```python
from build123d import *

# Parameters (mm, degrees)
F0_R     = 5
F1_DEPTH = 10
F2_SIZE  = 0.5
F4_D     = 9


with BuildPart() as f1:
    # F0 (on Front) → F1 (new body, symmetric)
    with BuildSketch(Plane.XZ):
        Polygon((18, 18), (0, 18), (-18, 18), (-18, -1), (-35, -1), (-35, -25), (0, -25), (35, -25), (35, -1), (18, -1), align=None)
        Circle(F0_R, mode=Mode.SUBTRACT)
    extrude(amount=F1_DEPTH, both=True)

    # F2
    f2_edges = [f1.edges().sort_by_distance(p)[0] for p in [
        (0, 10, 18),
        (-18, 0, 18),
        (0, -10, 18),
        (18, 0, 18),
        (-18, 0, -1),
        (-26.5, 10, -1),
        (-35, 0, -1),
        (-26.5, -10, -1),
        (-18, 10, 8.5),
        (-18, -10, 8.5),
        (-35, 10, -13),
        (-35, 0, -25),
        (-35, -10, -13),
        (35, 0, -25),
        (35, 10, -13),
        (35, 0, -1),
        (35, -10, -13),
        (18, 10, 8.5),
        (18, -10, 8.5),
        (18, 0, -1),
        (26.5, 10, -1),
        (26.5, -10, -1),
        (0, 10, -25),
        (0, -10, -25),
    ]]
    chamfer(f2_edges, length=F2_SIZE)

    # F4 (through all)
    with Locations(Plane(origin=(0, 0, -25), x_dir=(1, 0, 0), z_dir=(0, 0, -1))):
        with Locations((-26, 0), (26, 0)):
            Hole(F4_D / 2)


solid = f1.part
```
Geometry: final body of the model. Coordinates: model frame, mm. A direction names the side the tool comes from. Coordinates: 2 decimals unless noted, no trailing zeros. Order: outer loops, then holes, each group sorted by start corner. A loop starts at its lowest first (then second) coordinate and runs counter-clockwise, first axis right, second up. Notation, with made-up numbers: (-18, -2.5) - (4, -2.5) arc R29 cw to (4, 32.5) - close; hole circle Ø9 at (-23, -29.75). An arc over 180 degrees is marked (long way). Return JSON: item names as keys, results as strings. Group by question number.
1. Cut plane D-D (z = -14.5). Output: boundary loops of the cut face in (x, y), plus the area to 3 significant figures.
2. Pull-direction query (X, two-part tool) for faces 1 (the face through (0, 10, -8)), 2 (the face through (-18, 0, 9)), 3 (the face through (30.496, -0.198, -12.832)); classes: pulls with the +X half, pulls with the -X half, needs draft (parallel to the pull), parting line crosses it, or undercut.
3. Set-up query: faces 4 (the face through (-1.08, 0.14, -4.88)), 5 (the face through (-28.2, -4.4, -1)), 6 (the face through (18, 0, 8)). Return all of +Z, -Z, +X, -X, +Y, -Y with unobstructed straight access to the full face (end or side cutting, diameter ignored); none if empty.
4. Cut plane C-C (y = 8). Output: boundary loops of the cut face in (x, z).
5. Pin query (flat end, axial travel): pin 1 (9 mm diameter, centred on y = 2.5, z = 9.5, fed in from -X); pin 2 (1 mm diameter, centred on x = -19.5, y = 0.5, fed in from +Z); pin 3 (8 mm diameter, centred on x = 0, z = 0, fed in from +Y); pin 4 (9 mm diameter, centred on y = -3.5, z = 7, fed in from +X). Return the tip coordinate at first contact, or that it passes through.
6. Cut plane B-B (y = 0). Output: boundary loops of the cut face in (x, z), plus the area to 3 significant figures.
7. Material intervals for line 1 along Y through (x, z) = (26, -13); line 2 along X through (y, z) = (-4, -17); line 3 along X through (y, z) = (0.5, -20), sorted ascending. Write a range as [from, to].
8. Cut plane A-A (x = 26). Output: boundary loops of the cut face in (y, z), plus the area to 4 significant figures.
Resolved:
{
 "1": {"outline": "(-35, -9.5) - (-34.5, -10) - (34.5, -10) - (35, -9.5) - (35, 9.5) - (34.5, 10) - (-34.5, 10) - (-35, 9.5) - close; hole circle Ø9 at (-26, 0); hole circle Ø9 at (26, 0)", "area": "1,270 mm²"},
 "2": {"face 1": "needs draft", "face 2": "pulls with the -X half", "face 3": "undercut"},
 "3": {"face 4": "+Y, -Y", "face 5": "+Z, -X, +Y, -Y", "face 6": "+Z, +X, +Y, -Y"},
 "4": {"outline": "(-35, -24.5) - (-34.5, -25) - (34.5, -25) - (35, -24.5) - (35, -1.5) - (34.5, -1) - (18.5, -1) - (18, -0.5) - (18, 17.5) - (17.5, 18) - (-17.5, 18) - (-18, 17.5) - (-18, -0.5) - (-18.5, -1) - (-34.5, -1) - (-35, -1.5) - close; hole circle Ø10 at (0, 0)"},
 "5": {"pin 1": "stops at x = -18", "pin 2": "stops at z = -1", "pin 3": "passes through", "pin 4": "stops at x = 18"},
 "6": {"outline": "(-35, -24.5) - (-34.5, -25) - (-30.5, -25) - (-30.5, -1) - (-34.5, -1) - (-35, -1.5) - close; (-21.5, -25) - (21.5, -25) - (21.5, -1) - (18.5, -1) - (18, -0.5) - (18, 17.5) - (17.5, 18) - (-17.5, 18) - (-18, 17.5) - (-18, -0.5) - (-18.5, -1) - (-21.5, -1) - close; (30.5, -25) - (34.5, -25) - (35, -24.5) - (35, -1.5) - (34.5, -1) - (30.5, -1) - close; hole circle Ø10 at (0, 0)", "area": "1,850 mm²"},
 "7": {"line 1": "y = [-10, -4.5], [4.5, 10]", "line 2": "x = [-35, -28.06], [-23.94, 23.94], [28.06, 35]", "line 3": "x = [-35, -30.47], [-21.53, 21.53], [30.47, 35]"},
 "8": {"outline": "(-10, -24.5) - (-9.5, -25) - (-4.5, -25) - (-4.5, -1) - (-9.5, -1) - (-10, -1.5) - close; (4.5, -25) - (9.5, -25) - (10, -24.5) - (10, -1.5) - (9.5, -1) - (4.5, -1) - close", "area": "263.5 mm²"}
}
